Source: CAD feature listing. Evaluate the final solid. Frame: model axes, mm. A direction names the side the tool comes from. Coordinates: 2 decimals unless noted, no trailing zeros. Loops run counter-clockwise (first coordinate to the right, second up) from the corner with the lowest first, then second, coordinate; pieces in that order, holes last. Notation, with made-up numbers: M 30,-24.5 L 83,-24.5 A23 cw 83,12.5 Z; hole C 25.25,11.5 d4. An arc over 180 degrees is marked long. One line per question, with ' | ' between items. Start each with the question number.
1. Section query A-A, the plane x = 23. Output: boundary loops of the cut face in (y, z), and give its area (3 significant figures).
2. Ray query, probe 1 along Y at (x, z) = (41, 41.5); probe 2 along Y at (x, z) = (8.5, 136.5); probe 3 along Z at (x, y) = (43.5, 12). Return the intervals inside material, ascending.
3. Mould query, pull axis Z, two halves, no side actions, for faces 1 (the flat face through (34, 39.047, 79)), 2 (the flat face through (19.68, 25.97, 11.32)). Classes: pulls with the +Z half, pulls with the -Z half, needs draft (parallel to the pull), parting line crosses it, or undercut.
4. Pin query (flat end, axial travel): P1, Ø3.5, axis at x = 57, y = 10.5, coming from the +Z side; P2, Ø12, axis at y = 31.5, z = 87.5, coming from the +X side; P3, Ø0.8, axis at x = 22, z = 1.5, coming from the -Y side; P4, Ø10, axis at x = 9.5, z = 117.5, coming from the -Y side. Return the tip coordinate at first contact, or that it passes through.
5. Access query for faces 3 (the flat face through (23, 10, 2.002)), 4 (the flat face through (3.4, 36, 73)), 5 (the flat face through (27, 10, 3.782)). Directions: +Z, -Z, +X, -X, +Y, -Y. A direction counts if a zero-diameter tool reaches every point of the face in a straight line with its end or side. Return the directions, or none.
```python
from build123d import *

# Parameters (mm, degrees)
EXTRUDE_1_DEPTH = 69
SKETCH_7_W      = 3
SKETCH_7_H      = 1.8


with BuildPart() as part:
    # 草图2 → 凸台-拉伸1 (new body)
    with BuildSketch(Plane(origin=(0, 0, 0), x_dir=(0, 0, -1), z_dir=(1, 0, 0))):
        with BuildLine():
            Line((-2.001625282, 3.147074334), (-2.001625282, 17.164444968))
            Line((-2.001625282, 17.164444968), (-18.214026207, 37.447074334))
            Line((-18.214026207, 37.447074334), (-138.628938569, 37.447074334))
            ThreePointArc((-138.628938569, 37.447074334), (-141.499289796, 36.38190324), (-142.979906861, 33.70211244))
            Line((-142.979906861, 33.70211244), (-147.579966657, 3.147074334))
            Line((-147.579966657, 3.147074334), (-149.197997295, 3.147074334))
            Line((-149.197997295, 3.147074334), (-144.562077149, 33.940308116))
            ThreePointArc((-144.562077149, 33.940308116), (-142.543053879, 37.594568297), (-138.628938569, 39.047074334))
            Line((-138.628938569, 39.047074334), (-17.444620599, 39.047074334))
            Line((-17.444620599, 39.047074334), (-0.401625282, 17.725324466))
            Line((-0.401625282, 17.725324466), (-0.401625282, 3.147074334))
            Line((-0.401625282, 3.147074334), (-2.001625282, 3.147074334))
        make_face()
    extrude(amount=EXTRUDE_1_DEPTH)

    # 扫描1: sweep along a path in 草图17
    with BuildLine(Plane.ZY) as sweep_1_path:
        Line((147.579966657, 3.147074334), (143.056789207, 33.191435819))
        ThreePointArc((143.056789207, 33.191435819), (141.374269815, 36.236652636), (138.112507057, 37.447074334))
        Line((138.112507057, 37.447074334), (18.214026207, 37.447074334))
        Line((18.214026207, 37.447074334), (2.001625282, 17.164444968))
        Line((2.001625282, 17.164444968), (2.001625282, 3.147074334))
    # 草图7 → 扫描1 (sweep)
    with BuildSketch(Plane.XZ.offset(-3.147074334)):
        with Locations((34.5, 146.679966657)):
            Rectangle(SKETCH_7_W, SKETCH_7_H)
        with Locations((27.1, 146.679966657)):
            Rectangle(SKETCH_7_W, SKETCH_7_H)
        with Locations((19.7, 146.679966657)):
            Rectangle(SKETCH_7_W, SKETCH_7_H)
        with Locations((12.3, 146.679966657)):
            Rectangle(SKETCH_7_W, SKETCH_7_H)
        with Locations((4.9, 146.679966657)):
            Rectangle(SKETCH_7_W, SKETCH_7_H)
        with Locations((41.9, 146.679966657)):
            Rectangle(SKETCH_7_W, SKETCH_7_H)
        with Locations((49.3, 146.679966657)):
            Rectangle(SKETCH_7_W, SKETCH_7_H)
        with Locations((56.7, 146.679966657)):
            Rectangle(SKETCH_7_W, SKETCH_7_H)
        with Locations((64.1, 146.679966657)):
            Rectangle(SKETCH_7_W, SKETCH_7_H)
    sweep(path=sweep_1_path.line, transition=Transition.RIGHT)


solid = part.part
```
Taken from the geometry:
1) outline: M 3.15,0.4 L 17.73,0.4 L 39.05,17.44 L 39.05,138.63 A6 ccw 33.94,144.56 L 3.15,149.2 L 3.15,147.58 L 33.7,142.98 A4.4 cw 37.45,138.63 L 37.45,18.21 L 17.16,2 L 3.15,2 Z | area: 320 mm^2
2) probe 1: 35.67 to 39.05 | probe 2: 37.45 to 39.05 | probe 3: 0.4 to 2, 146.25 to 147.87
3) face 1: needs draft | face 2: undercut
4) P1: z = 148.35 | P2: x = 69 | P3: y = 3.15 | P4: y = 35.67
5) face 3: -Y | face 4: -X, -Y | face 5: +X, -X, -Y
